Can you work these out from the drawing? Everything is in mm from the part's minimum corner. A direction names the side the tool comes from. Give positions to 0.01 mm unless a question says otherwise; leave off trailing zeros. Order: outer loops, then holes, each group sorted by start corner. A loop starts at its lowest first (then second) coordinate and runs counter-clockwise, first axis right, second up. Notation, with made-up numbers: M 42,85 L 49,85 A25 cw 49,124 Z; hole C 4,-2 d11. An arc over 180 degrees is marked long. Answer as a JSON object with one key per item and string values.
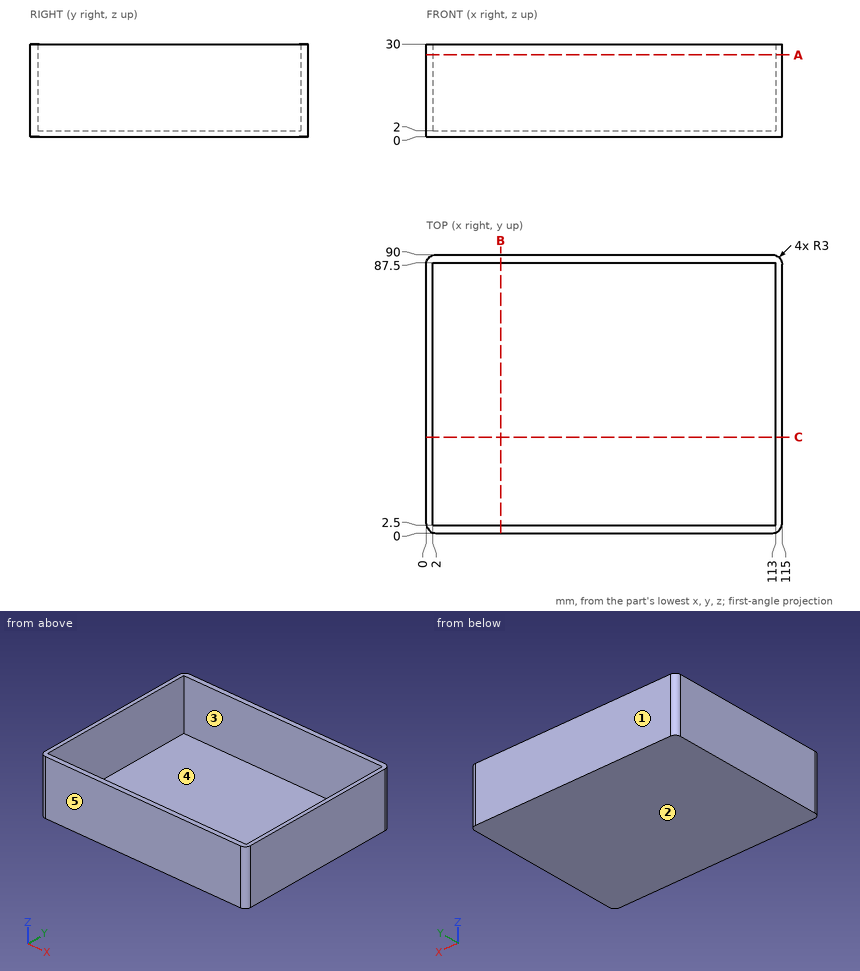
1) For the marked faces 4 and 5, which set-ups out of +Z, -Z, +X, -X, +Y, -Y let a thin tool reach every point of the face, with its end or its side?
Results found:
{"face 4": "+Z", "face 5": "+Z, -Z, +X, -X, -Y"}
2) I want a section at A-A on z = 26.5. Write out the boundary of the cut face in (x, y), and give its area (3 significant figures).
Results found:
{"outline": "M 0,3 A3 ccw 3,0 L 112,0 A3 ccw 115,3 L 115,87 A3 ccw 112,90 L 3,90 A3 ccw 0,87 Z; hole M 2,2.5 L 113,2.5 L 113,87.5 L 2,87.5 Z", "area": "907 mm²"}
3) I'm going to push a flat-ended pin straight in: pin 1 Ø6 at (x, y) = (50.5, 77) entering from +Z. Where does the tip first touch, or does it pass through?
Results found:
{"pin 1": "stops at z = 2"}
4) I want a section at B-B on x = 24. Write out the boundary of the cut face in (y, z), and give its area (3 significant figures).
Results found:
{"outline": "M 0,0 L 90,0 L 90,30 L 87.5,30 L 87.5,2 L 2.5,2 L 2.5,30 L 0,30 Z", "area": "320 mm²"}
5) I want a section at C-C on y = 31. Write out the boundary of the cut face in (x, z).
Results found:
{"outline": "M 0,0 L 115,0 L 115,30 L 113,30 L 113,2 L 2,2 L 2,30 L 0,30 Z"}
6) I need wall thicknesses on L1, parallel to Y at x = 110, z = 23.5; L2, parallel to X at y = 27.5, z = 21.5; L3, parallel to Z at x = 92, y = 6. Which ranges of each line are inside material? Lowest first, please.
Results found:
{"L1": "y = 0 to 2.5, 87.5 to 90", "L2": "x = 0 to 2, 113 to 115", "L3": "z = 0 to 2"}
7) Thinking about a two-plate mould opening in Y: for the marked faces 1, 2 and 3, which applies, pulls with the +Y half, pulls with the -Y half, needs draft (parallel to the pull), parting line crosses it, or undercut?
Results found:
{"face 1": "pulls with the +Y half", "face 2": "needs draft", "face 3": "undercut"}
